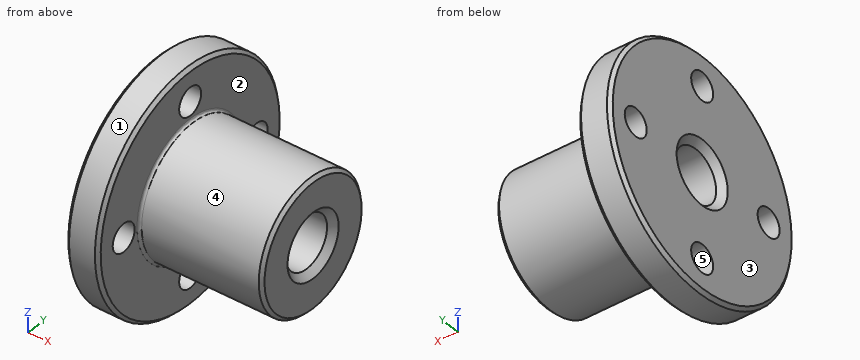
```python
from build123d import *

# Parameters (mm, degrees)
SKETCH1_W                      = 5
SKETCH1_H                      = 18
SKETCH2_R                      = 10
BOSS_EXTRUDE1_DEPTH            = 19
F_4_3_4_3_DIAMETER_HOLE1_D     = 4.3
F_4_3_4_3_DIAMETER_HOLE1_DEPTH = 24
F_8_0_8_DIAMETER_HOLE1_D       = 8
CHAMFER1_SIZE                  = 0.5
CHAMFER2_SIZE                  = 1
FILLET1_R                      = 0.4


with BuildPart() as part:
    # Sketch1 → Revolve1 (revolve)
    with BuildSketch(Plane.XY, mode=Mode.PRIVATE) as revolve1_sk:
        with Locations((2.5, 9)):
            Rectangle(SKETCH1_W, SKETCH1_H)
    revolve(revolve1_sk.sketch.rotate(Axis((0, 0, 0), (1, 0, 0)), 270), axis=Axis((0, 0, 0), (1, 0, 0)))

    # Sketch2 → Boss-Extrude1 (add)
    with BuildSketch(Plane(origin=(5, 0, 0), x_dir=(0, 0, -1), z_dir=(1, 0, 0))):
        Circle(SKETCH2_R)
    extrude(amount=BOSS_EXTRUDE1_DEPTH)

    # Ø4.3 (4.3) Diameter Hole1
    with Locations(Plane.ZY):
        with Locations((0, 13), (0, -13), (-13, 0), (13, 0)):
            Hole(F_4_3_4_3_DIAMETER_HOLE1_D / 2, depth=F_4_3_4_3_DIAMETER_HOLE1_DEPTH)

    # Ø8.0 (8) Diameter Hole1 (through all)
    with Locations(Plane(origin=(24, 0, 0), x_dir=(0, 0, -1), z_dir=(1, 0, 0))):
        with Locations((0, 0)):
            Hole(F_8_0_8_DIAMETER_HOLE1_D / 2)

    # Chamfer1
    chamfer1_edges = [part.edges().sort_by_distance(p)[0] for p in [
        (5, 0, 18),
        (0, 0, 18),
        (24, 0, 10),
    ]]
    chamfer(chamfer1_edges, length=CHAMFER1_SIZE)

    # Chamfer2
    chamfer2_edges = [part.edges().sort_by_distance(p)[0] for p in [
        (24, 0, -4),
        (0, 0, -4),
    ]]
    chamfer(chamfer2_edges, length=CHAMFER2_SIZE)

    # Fillet1
    fillet1_edges = [part.edges().sort_by_distance(p)[0] for p in [
        (5, 0, 10),
    ]]
    fillet(fillet1_edges, radius=FILLET1_R)


solid = part.part
```
CAD build for the part. Positions are in the model's coordinates, mm. Face numbers are marked on the shaded views. A direction names the side the tool comes from. Round coordinates to 2 decimals unless told otherwise and drop trailing zeros. Order: outer loops, then holes, each group sorted by start corner. A loop starts at its lowest first (then second) coordinate and runs counter-clockwise, first axis right, second up.
Item 1: Mould opens along Y. For the marked faces 3, 4 and 5 say: pulls with the +Y half, pulls with the -Y half, needs draft (parallel to the pull), parting line crosses it, or undercut.
Item 2: Saw through at C-C on x = 8.25. Write the cut outline in (y, z), then the cut area to 3 significant figures.
Item 3: Saw through at A-A on y = 0. State how many separate pieces and enclosed holes the cut face has, then the cut area to 3 significant figures.
Item 4: Tool access for the marked faces 1 and 2: list every direction of +Z, -Z, +X, -X, +Y, -Y with a clear straight run to the whole face (end or side of a thin tool).
Item 5: Pin check, flat tips, straight feed: pin 1 (12 mm diameter, centred on x = 4, y = -11, fed in from +Z); pin 2 (5 mm diameter, centred on y = 13, z = 0, fed in from +X); pin 3 (12 mm diameter, centred on x = 7, z = 12, fed in from -Y); pin 4 (1 mm diameter, centred on x = 20.5, z = 12, fed in from -Y). Stop position of each tip, or through.
Item 6: Probe line 1 along Y through (x, z) = (1.35, 0); line 2 along Z through (x, y) = (4.5, 0.5); line 3 along X through (y, z) = (-12.5, 10). List the from-to ranges inside material, lowest first.
Reported:
1. face 3: needs draft
1. face 4: parting line crosses it
1. face 5: undercut
2. outline: circle Ø20 at (0, 0); hole circle Ø8 at (0, 0)
2. area: 264 mm2
3. separate pieces: 4
3. enclosed holes: 0
3. area: 322 mm2
4. face 1: +X, -X
4. face 2: +X
5. pin 1: stops at z = 17.29
5. pin 2: stops at x = 5
5. pin 3: stops at y = -16.77
5. pin 4: passes through
6. line 1: y = -18 to -15.15, -10.85 to -4, 4 to 10.85, 15.15 to 18
6. line 2: z = -17.99 to -15.09, -10.91 to -3.97, 3.97 to 10.91, 15.09 to 17.99
6. line 3: x = 0 to 5
